```python
from build123d import *

# Parameters (mm, degrees)
F0_W     = 144.836355
F0_H     = 89.3826
F2_DEPTH = 25.4
F3_DEPTH = 25.401


with BuildPart() as f2:
    # F0 (on Top) → F2 (new body)
    with BuildSketch(Plane.XY):
        with Locations((-11.173098, 0.619659)):
            Rectangle(F0_W, F0_H)
    extrude(amount=F2_DEPTH)

    # F1 (on Top) → F3 (cut, through all)
    with BuildSketch(Plane.XY):
        with BuildLine():
            ThreePointArc((-65.383278, 6.35), (-71.733278, 0), (-65.383278, -6.35))
            Line((-65.383278, -6.35), (44.27854, -6.35))
            ThreePointArc((44.27854, -6.35), (50.62854, 0), (44.27854, 6.35))
            Line((44.27854, 6.35), (-65.383278, 6.35))
        make_face()
    extrude(amount=F3_DEPTH, mode=Mode.SUBTRACT)


solid = f2.part
```
Design review of the part built by this model. Coordinates are the model's own, in mm. A direction names the side the tool comes from. Give positions to 0.01 mm unless a question says otherwise; leave off trailing zeros. Write each loop counter-clockwise with the first axis right and the second up, starting at its lowest first coordinate (ties: lowest second). Pieces come first, ordered by that corner, then holes. Notation, with made-up numbers: (44, 54) -> (83, 54) arc R32 ccw to (83, 88) -> close; hole circle Ø10 at (6.25, 87). An arc over 180 degrees is marked (long way). Answer in a Markdown table with one row per item.
(1) Consider section A-A (y = 0). State the section outline as (x, z) points.
Results:
| item | result |
|---|---|
| outline | (-83.59, 0) -> (-71.73, 0) -> (-71.73, 25.4) -> (-83.59, 25.4) -> close; (50.63, 0) -> (61.25, 0) -> (61.25, 25.4) -> (50.63, 25.4) -> close |
(2) To check wall thickness, follow probe 1 along Y at (x, z) = (9.5, 5.75); probe 2 along X at (y, z) = (-1, 9.5). State the ranges of each line that lie inside material, in increasing order.
Results:
| item | result |
|---|---|
| probe 1 | -44.07 to -6.35, 6.35 to 45.31 |
| probe 2 | -83.59 to -71.65, 50.55 to 61.25 |
(3) Consider section C-C (z = 23.75). State the section outline as (x, y) points.
Results:
| item | result |
|---|---|
| outline | (-83.59, -44.07) -> (61.25, -44.07) -> (61.25, 45.31) -> (-83.59, 45.31) -> close; hole (-65.38, -6.35) -> (44.28, -6.35) arc R6.35 ccw to (44.28, 6.35) -> (-65.38, 6.35) arc R6.35 ccw to start |
(4) Mouldability with a two-part tool opening along Y and no side actions: class faces 1 (the flat face through (-12, 11, 0)), 2 (the flat face through (-12, 45.311, 13)), 3 (the flat face through (-10, 6.35, 13)) as +Y half, -Y half, draft (parallel to the pull), parting line (faces both ways), or undercut.
Results:
| item | result |
|---|---|
| face 1 | draft |
| face 2 | +Y half |
| face 3 | undercut |
(5) Consider section B-B (x = -6.5). State the section outline as (y, z) points, then the cut area to 3 significant figures.
Results:
| item | result |
|---|---|
| outline | (-44.07, 0) -> (-6.35, 0) -> (-6.35, 25.4) -> (-44.07, 25.4) -> close; (6.35, 0) -> (45.31, 0) -> (45.31, 25.4) -> (6.35, 25.4) -> close |
| area | 1,950 mm2 |
(6) For faces 4 (the cylindrical face through (50.627, -0.14, 12.522)), 5 (the flat face through (-12, 11, 25.4)), list the 3-axis set-ups (+Z, -Z, +X, -X, +Y, -Y) from which the entire face can be reached by the end or side of a thin tool; tool diameter is ignored.
Results:
| item | result |
|---|---|
| face 4 | +Z, -Z |
| face 5 | +Z, +X, -X, +Y, -Y |
